The model under review builds one solid part; all positions refer to its coordinate system, in mm. A direction names the side the tool comes from. Give positions to 0.01 mm unless a question says otherwise; leave off trailing zeros. Loops run counter-clockwise (first coordinate to the right, second up) from the corner with the lowest first, then second, coordinate; pieces in that order, holes last. Notation, with made-up numbers: M -8,64 L 44,64 A28 cw 44,99 Z; hole C 36.5,50.5 d3. An arc over 180 degrees is marked long. One line per item, written item: value. Start each with the question number.
Q1. For pin 1 (3 mm diameter, centred on y = 3.5, z = 7.5, fed in from +X); pin 2 (6 mm diameter, centred on y = 5.5, z = 16.5, fed in from -X); pin 3 (6 mm diameter, centred on x = -1, y = 0.5, fed in from -Z), all flat-tipped, find the tip position at first contact; note any pin that passes through.
Q2. We need section C-C on z = 20.5. Write out the cut boundary in (x, y).
Q3. For faces 4 (the face through (-4.919, -7.715, 2.028)), 5 (the face through (3.48, -1.1, 7.42)), list the 3-axis set-ups (+Z, -Z, +X, -X, +Y, -Y) from which the entire face can be reached by the end or side of a thin tool; tool diameter is ignored.
Q4. We need section D-D on z = 6.75. Write out the cut boundary in (x, y), plus the area to 3 significant figures.
Q5. Mouldability with a two-part tool opening along Y and no side actions: class faces 1 (the face through (-4, 2, 0)), 2 (the face through (0.9, 4.05, 16.34)), 3 (the face through (4.006, 1.262, 0.986)) as released by +Y, released by -Y, zero draft, split by the parting line, or undercut.
Q6. We need section A-A on y = 0. Write out the cut boundary in (x, z).
Q7. To check wall thickness, follow line 1 along X through (y, z) = (0, 17.75); line 2 along X through (y, z) = (0, 10); line 3 along Y through (x, z) = (-1.25, 16). State the ranges of each line that lie inside material, in increasing order. Write a range as from..to.
```python
from build123d import *

# Parameters (mm, degrees)
F0_W        = 5
F0_H        = 4
F2_R        = 4.2
F2_R_2      = 3.65
F3_DEPTH    = 2
F3_FACE_R   = 3.65
F3_FACE_R_2 = 2.65
F4_DEPTH    = 13


with BuildPart() as f1:
    # F0 (on Front) → F1 (revolve)
    with BuildSketch(Plane.XZ):
        Polygon((-4.15, 0), (-2.65, 0), (-2.65, 24), (-4.15, 24), (-4.15, 8.898979), (-4.15, 4), align=None)
        with Locations((-6.65, 2)):
            Rectangle(F0_W, F0_H)
        Polygon((-9.15, 4), (-4.15, 4), (-4.15, 8.898979), align=None)
    revolve(axis=Axis((0, 0, 13.376878), (0, 0, 1)))

    # F2 (on Top) → F3 (cut)
    with BuildSketch(Plane.XY):
        Circle(F2_R)
        Circle(F2_R_2, mode=Mode.SUBTRACT)
    extrude(amount=F3_DEPTH, mode=Mode.SUBTRACT)

    # F3_face (on face) → F4 (cut)
    with BuildSketch(Plane(origin=(0, 0, 0), x_dir=(1, 0, 0), z_dir=(0, 0, -1))):
        Circle(F3_FACE_R)
        Circle(F3_FACE_R_2, mode=Mode.SUBTRACT)
    extrude(amount=-F4_DEPTH, mode=Mode.SUBTRACT)


solid = f1.part
```
Solved:
1. pin 1: x = 6.35
1. pin 2: x = -3.31
1. pin 3: z = 2
2. outline: C 0,0 d8.3; hole C 0,0 d5.3
3. face 4: +Z, -Z
3. face 5: -Z
4. outline: C 0,0 d12.69; hole C 0,0 d7.3
4. area: 84.6 mm2
5. face 1: zero draft
5. face 2: split by the parting line
5. face 3: undercut
6. outline: M -9.15,0 L -4.2,0 L -4.2,2 L -3.65,2 L -3.65,13 L -2.65,13 L -2.65,24 L -4.15,24 L -4.15,8.9 L -9.15,4 Z; M 2.65,13 L 3.65,13 L 3.65,2 L 4.2,2 L 4.2,0 L 9.15,0 L 9.15,4 L 4.15,8.9 L 4.15,24 L 2.65,24 Z
7. line 1: -4.15..-2.65, 2.65..4.15
7. line 2: -4.15..-3.65, 3.65..4.15
7. line 3: -3.96..-2.34, 2.34..3.96
